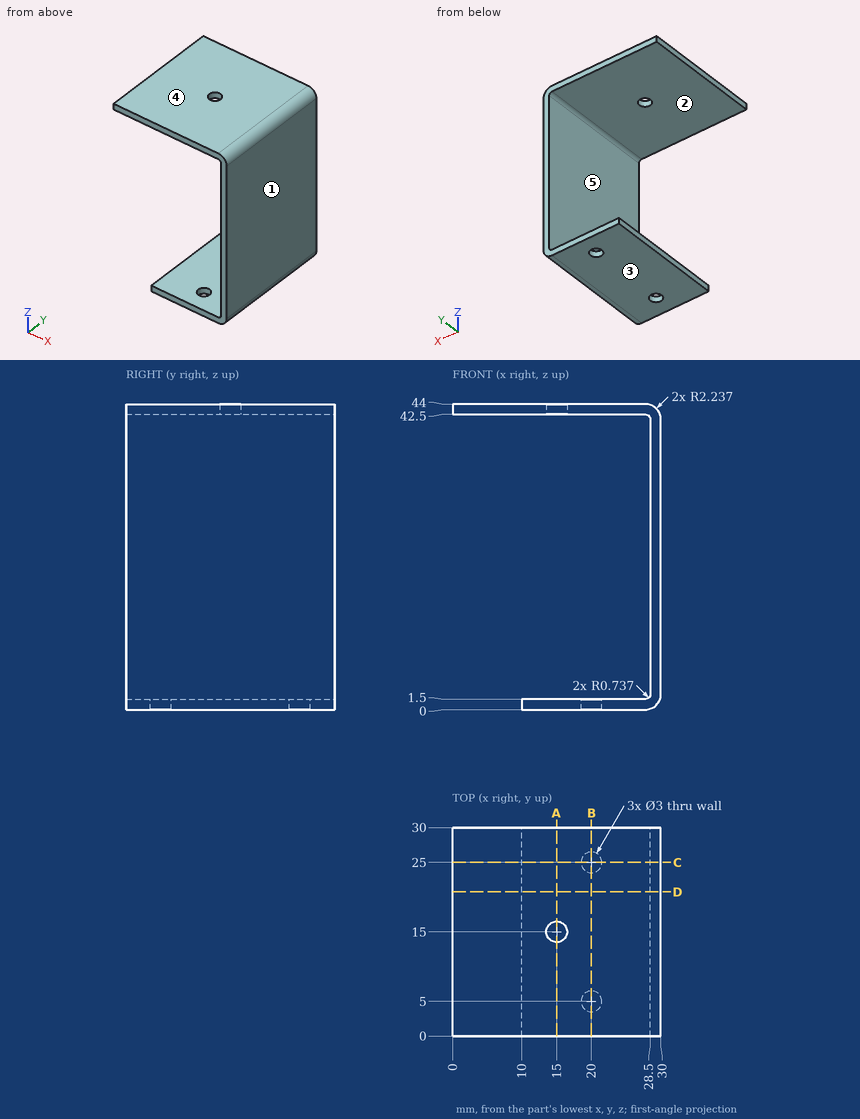
Geometry check sheet. Reference: drawing and pictorial views, mm from the part's lowest x, y, z. A direction names the side the tool comes from. Round coordinates to 2 decimals unless told otherwise and drop trailing zeros. Order: outer loops, then holes, each group sorted by start corner. A loop starts at its lowest first (then second) coordinate and runs counter-clockwise, first axis right, second up. Notation, with made-up numbers: (-37, 61) - (17, 61) arc R24 ccw to (17, 95) - close; hole circle Ø10 at (-31.75, -12). An arc over 180 degrees is marked (long way). Write item = value, one per line.
Q1. Section check B-B (x = 20). Record the boundary of the cut face in (y, z).
Computed:
outline = (0, 0) - (3.5, 0) - (3.5, 1.5) - (0, 1.5) - close; (0, 42.5) - (30, 42.5) - (30, 44) - (0, 44) - close; (6.5, 0) - (23.5, 0) - (23.5, 1.5) - (6.5, 1.5) - close; (26.5, 0) - (30, 0) - (30, 1.5) - (26.5, 1.5) - close
Q2. Section check A-A (x = 15). Record the boundary of the cut face in (y, z).
Computed:
outline = (0, 0) - (30, 0) - (30, 1.5) - (0, 1.5) - close; (0, 42.5) - (13.5, 42.5) - (13.5, 44) - (0, 44) - close; (16.5, 42.5) - (30, 42.5) - (30, 44) - (16.5, 44) - close
Q3. Thickness scan on line 1 along Y through (x, z) = (20, 1.05); line 2 along Z through (x, y) = (23.25, 23); line 3 along Y through (x, z) = (15, 43). Record the ranges inside material, lowest first.
Computed:
line_1 = 0 to 3.5, 6.5 to 23.5, 26.5 to 30
line_2 = 0 to 1.5, 42.5 to 44
line_3 = 0 to 13.5, 16.5 to 30
Q4. Section check D-D (y = 20.75). Record the boundary of the cut face in (x, z).
Computed:
outline = (0, 42.5) - (27.76, 42.5) arc R0.74 cw to (28.5, 41.76) - (28.5, 2.24) arc R0.74 cw to (27.76, 1.5) - (10, 1.5) - (10, 0) - (27.76, 0) arc R2.24 ccw to (30, 2.24) - (30, 41.76) arc R2.24 ccw to (27.76, 44) - (0, 44) - close
Q5. Draft check along Z on the marked faces 1, 2 and 3. Enter one of: pulls with the +Z half, pulls with the -Z half, needs draft (parallel to the pull), parting line crosses it, or undercut.
Computed:
face_1 = needs draft
face_2 = undercut
face_3 = pulls with the -Z half
Q6. Go/stop test with flat-tipped pins: pin 1 (0.8 mm diameter, centred on y = 18, z = 0.5, fed in from -X); pin 2 (1 mm diameter, centred on y = 8, z = 25.5, fed in from -X). Record where each tip stops, or that it passes through.
Computed:
pin_1 = 10
pin_2 = 28.5
Q7. Section check C-C (y = 25). Record the boundary of the cut face in (x, z).
Computed:
outline = (0, 42.5) - (27.76, 42.5) arc R0.74 cw to (28.5, 41.76) - (28.5, 2.24) arc R0.74 cw to (27.76, 1.5) - (21.5, 1.5) - (21.5, 0) - (27.76, 0) arc R2.24 ccw to (30, 2.24) - (30, 41.76) arc R2.24 ccw to (27.76, 44) - (0, 44) - close; (10, 0) - (18.5, 0) - (18.5, 1.5) - (10, 1.5) - close
Q8. Tool access check on the marked faces 4 and 5. Record the directions out of +Z, -Z, +X, -X, +Y, -Y that give a thin tool (end or side, any length) a straight path to the whole face; none if there is none.
Computed:
face_4 = +Z, +X, -X, +Y, -Y
face_5 = -X, +Y, -Y
